```python
from build123d import *

# Parameters (mm, degrees)
F0_W        = 1400
F0_H        = 600
F0_W_2      = 1080
F0_H_2      = 280
F1_DEPTH    = 420
F1_FACE_W   = 1400
F1_FACE_H   = 600
F1_FACE_W_2 = 1080
F1_FACE_H_2 = 280
F2_DEPTH    = 80


with BuildPart() as f1:
    # F0 (on Front) → F1 (new body)
    with BuildSketch(Plane.XZ):
        with Locations((700, 300)):
            Rectangle(F0_W, F0_H)
        with Locations((700, 300)):
            Rectangle(F0_W_2, F0_H_2, mode=Mode.SUBTRACT)
    extrude(amount=F1_DEPTH)

    # F1_face (on face) → F2 (join)
    with BuildSketch(Plane(origin=(700, -420, 300), x_dir=(1, 0, 0), z_dir=(0, -1, 0))):
        Rectangle(F1_FACE_W, F1_FACE_H)
        Rectangle(F1_FACE_W_2, F1_FACE_H_2, mode=Mode.SUBTRACT)
    extrude(amount=F2_DEPTH)


solid = f1.part
```
Source: CAD feature listing. Evaluate the final solid. Frame: model axes, mm. A direction names the side the tool comes from. Coordinates: 2 decimals unless noted, no trailing zeros. Loops run counter-clockwise (first coordinate to the right, second up) from the corner with the lowest first, then second, coordinate; pieces in that order, holes last. Notation, with made-up numbers: M -20,49.5 L -2,49.5 A23 ccw -2,67.5 Z; hole C 33,-21 d10. An arc over 180 degrees is marked long. Use CSV: the item, a comma, the result in double quotes.
(1) Cut plane B-B on z = 424.5. Return loops of the section in (x, y).
Answers follow:
outline,"M 0,-500 L 160,-500 L 160,0 L 0,0 Z; M 1240,-500 L 1400,-500 L 1400,0 L 1240,0 Z"
(2) Reachability of faces 5 (the face through (690, -246, 0)), 6 (the face through (692, -246, 160)) from +Z, -Z, +X, -X, +Y, -Y: full face, straight path, thin tool, end or side. Return the list, or none.
Answers follow:
face 5,"-Z, +X, -X, +Y, -Y"
face 6,"+Y, -Y"
(3) Line query: line 1 (X direction, y = -254.5, z = 175); line 2 (Z direction, x = 747, y = -208.5). Output: solid intervals per line, ascending. Write a range as [from, to].
Answers follow:
line 1,"[0, 160], [1240, 1400]"
line 2,"[0, 160], [440, 600]"
(4) Cut plane A-A on x = 794.5. Return loops of the section in (y, z), and give its area (3 significant figures).
Answers follow:
outline,"M -500,0 L 0,0 L 0,160 L -500,160 Z; M -500,440 L 0,440 L 0,600 L -500,600 Z"
area,"160,000 mm²"
(5) Draft query along X for faces 1 (the face through (690, -246, 600)), 2 (the face through (1240, -246, 298)), 3 (the face through (1400, -246, 296)), 4 (the face through (0, -246, 296)). Return one class per face: pulls with the +X half, pulls with the -X half, needs draft (parallel to the pull), parting line crosses it, or undercut.
Answers follow:
face 1,"needs draft"
face 2,"undercut"
face 3,"pulls with the +X half"
face 4,"pulls with the -X half"
(6) Cut plane C-C on y = -165.5. Return loops of the section in (x, z).
Answers follow:
outline,"M 0,0 L 1400,0 L 1400,600 L 0,600 Z; hole M 160,160 L 1240,160 L 1240,440 L 160,440 Z"
